Can you work these out from the model? Positions are in its coordinate system, mm. A direction names the side the tool comes from. Coordinates: 2 decimals unless noted, no trailing zeros. Loops run counter-clockwise (first coordinate to the right, second up) from the corner with the lowest first, then second, coordinate; pieces in that order, holes last. Notation, with made-up numbers: (3.25, -32) - (19.25, -32) arc R10 cw to (19.25, -26) - close; hole circle Ø3 at (-3.75, 38.5). An arc over 180 degrees is marked (long way). Put each result on its own line as item: value. Start each with the question number.
from build123d import *

# Parameters (mm, degrees)
BOSS_EXTRUDE1_DEPTH = 20
FILLET1_R           = 20
FILLET2_R           = 20
SKETCH2_R           = 3
CUT_EXTRUDE2_DEPTH  = 40


with BuildPart() as part:
    # Sketch1 → Boss-Extrude1 (new, symmetric)
    with BuildSketch(Plane(origin=(0, 0, 0), x_dir=(1, 0, 0), z_dir=(0, 1, 0))):
        Polygon((-4.418120101, 15.201487277), (0.581879899, 15.201487277), (0.581879899, -29.798512723), (-24.418120101, -29.798512723), (-24.418120101, -24.798512723), (-4.418120101, -24.798512723), align=None)
    extrude(amount=BOSS_EXTRUDE1_DEPTH, both=True)

    # Fillet1
    fillet1_edges = [part.edges().sort_by_distance(p)[0] for p in [
        (-1.918120101, -20, -15.201487277),
    ]]
    fillet(fillet1_edges, radius=FILLET1_R)

    # Fillet2
    fillet2_edges = [part.edges().sort_by_distance(p)[0] for p in [
        (-1.918120101, 20, -15.201487277),
    ]]
    fillet(fillet2_edges, radius=FILLET2_R - 0.0001)  # a hair under: the kernel refuses the full size

    # Sketch2 → Cut-Extrude2 (cut)
    with BuildSketch(Plane.ZY.offset(4.418120101)):
        with Locations((4.798512723, 0)):
            Circle(SKETCH2_R)
    extrude(amount=-CUT_EXTRUDE2_DEPTH, mode=Mode.SUBTRACT)


solid = part.part
Q1. Please list where these lines run through material, in increasing order: line 1 along X through (y, z) = (3, -6); line 2 along Y through (x, z) = (-0.5, 6); line 3 along Z through (x, y) = (-12.75, 12). Write a range as [from, to].
Q2. On a 3-axis mill with a long thin cutter (end or side, diameter ignored), from which of +Z, -Z, +X, -X, +Y, -Y can I reach the whole of each face in a straight line? I mean faces 5 (the flat face through (0.582, 0, 12)), 6 (the flat face through (-15, 0, 24.799)). Say none if no direction works.
Q3. We'd pull the mould along Z, two halves only. Please class faces 1 (the flat face through (-3, -20, 23)), 2 (the cylindrical face through (-1.95, -1.15, 7.57)), 3 (the cylindrical face through (-1.883, -13.986, -9.498)), 4 (the flat face through (-12, 0, 29.799)): released by +Z, released by -Z, zero draft, split by the parting line, or undercut.
Q4. I want a section at A-A on y = 10.5. List the corners of the cut face in (x, z) for me, and give its area (3 significant figures).
Q5. Will these pins go through, and if not, where does the flat tip stop? pin 1 (10 mm diameter, centred on y = -14, z = -5, fed in from -X); pin 2 (5 mm diameter, centred on y = 0, z = 4.8, fed in from -X); pin 3 (12 mm diameter, centred on x = -7, y = -7.5, fed in from -Z); pin 4 (6 mm diameter, centred on x = -10, y = -7.5, fed in from -Z).
Q6. I want a section at B-B on x = -14.75. List the corners of the cut face in (y, z) for me.
Q7. I want a section at C-C on z = -5. List the corners of the cut face in (x, y) for me.
Q8. I want a section at D-D on y = -7.5. List the corners of the cut face in (x, z) for me, and give its area (3 significant figures).
Calculated:
1. line 1: [-4.42, 0.58]
1. line 2: [-20, -2.75], [2.75, 20]
1. line 3: [24.8, 29.8]
2. face 5: +Z, -Z, +X, +Y, -Y
2. face 6: -Z, -X, +Y, -Y
3. face 1: zero draft
3. face 2: undercut
3. face 3: released by -Z
3. face 4: released by +Z
4. outline: (-24.42, 24.8) - (-4.42, 24.8) - (-4.42, -12.22) - (0.58, -12.22) - (0.58, 29.8) - (-24.42, 29.8) - close
4. area: 310 mm2
5. pin 1: x = -4.42
5. pin 2: through
5. pin 3: z = -15.09
5. pin 4: z = 24.8
6. outline: (-20, 24.8) - (20, 24.8) - (20, 29.8) - (-20, 29.8) - close
7. outline: (-4.42, -17.44) - (0.58, -17.44) - (0.58, 17.44) - (-4.42, 17.44) - close
8. outline: (-24.42, 24.8) - (-4.42, 24.8) - (-4.42, -13.74) - (0.58, -13.74) - (0.58, 29.8) - (-24.42, 29.8) - close
8. area: 318 mm2
